Geometry: final body of the model. Coordinates: model frame, mm. A direction names the side the tool comes from. Coordinates: 2 decimals unless noted, no trailing zeros. Write each loop counter-clockwise with the first axis right and the second up, starting at its lowest first coordinate (ties: lowest second). Pieces come first, ordered by that corner, then holes. Notation, with made-up numbers: (-5.75, -30) -> (38.25, -30) arc R19 ccw to (38.25, 3) -> close; hole circle Ø10 at (71.5, 15). An arc over 180 degrees is marked (long way). One line per item, written item: value.
```python
from build123d import *

# Parameters (mm, degrees)
F1_DEPTH = 6
F2_SIZE  = 1
F3_W     = 12
F3_H     = 23
F4_DEPTH = 1
F5_COUNT = 4
F6_R     = 1
F7_DEPTH = 25


with BuildPart() as f1:
    # F0 (on Top) → F1 (new body)
    with BuildSketch(Plane.XY):
        with BuildLine():
            Line((11.3636297451, -30.5553255426), (-11.5303793462, 30.4927918061))
            ThreePointArc((-11.5303793462, 30.4927918061), (-30.524172541, -11.4470472475), (11.3636297451, -30.5553255426))
        make_face()
        with BuildLine():
            ThreePointArc((11.3636297451, -30.5553255426), (26.7695193241, -18.6051830186), (32.6, 0))
            ThreePointArc((32.6, 0), (18.5319944058, 26.8202383163), (-11.5303793462, 30.4927918061))
            Line((-11.5303793462, 30.4927918061), (11.3636297451, -30.5553255426))
        make_face()
    extrude(amount=F1_DEPTH)

    # F2
    f2_edges = [f1.edges().sort_by_distance(p)[0] for p in [
        (-11.36363, 30.555326, 6),
        (-11.36363, 30.555326, 0),
    ]]
    chamfer(f2_edges, length=F2_SIZE)

    # F3 (on Front) → F4 (join, symmetric)
    with BuildSketch(Plane.XZ):
        with Locations((-26.536149025, 14.6011034735)):
            Rectangle(F3_W, F3_H)
    extrude(amount=F4_DEPTH, both=True)

    # F5: F1 ×4 about axis
    f5_axis = Axis((0, 0, 5), (0, 0, -1))


with BuildPart() as f1_1:
    add(f1.part)
    for i in range(1, F5_COUNT):
        add(f1.part.rotate(f5_axis, i * 360 / F5_COUNT))

    # F6 (on Top) → F7 (cut)
    with BuildSketch(Plane.XY):
        with Locations((-29.5159034431, -2.5976577308)):
            Circle(F6_R)
        with Locations((29.5159034431, 2.5976577308)):
            Circle(F6_R)
    extrude(amount=F7_DEPTH, mode=Mode.SUBTRACT)


solid = f1_1.part
```
(1) Section B-B (y = 0). Return the cut outline in (x, z).
Responses:
outline: (-32.6, 1) -> (-31.6, 0) -> (31.6, 0) -> (32.6, 1) -> (32.6, 5) -> (32.54, 5.06) -> (32.54, 26.1) -> (20.54, 26.1) -> (20.54, 6) -> (-20.54, 6) -> (-20.54, 26.1) -> (-32.54, 26.1) -> (-32.54, 5.06) -> (-32.6, 5) -> close
(2) Pull-direction query (X, two-part tool) for faces 1 (the flat face through (-27, 0, 26.101)), 2 (the flat face through (1, 27, 16)), 3 (the flat face through (-20.536, 0, 16)); classes: released by +X, released by -X, zero draft, split by the parting line, or undercut.
Responses:
face 1: zero draft
face 2: released by +X
face 3: undercut
(3) Reachability of faces 4 (the flat face through (0, 27, 26.101)), 5 (the flat face through (0, 32.536, 15)), 6 (the flat face through (0, 0, 0)), 7 (the flat face through (32.536, 0, 15)), 8 (the flat face through (0, 20.536, 16)) from +Z, -Z, +X, -X, +Y, -Y: full face, straight path, thin tool, end or side. Return the list, or none.
Responses:
face 4: +Z, +X, -X, +Y, -Y
face 5: +Z, +X, -X, +Y
face 6: -Z, +X, -X, +Y, -Y
face 7: +Z, +X, +Y, -Y
face 8: +Z, +X, -X
(4) Line query: line 1 (Z direction, x = -3, y = 19); line 2 (X direction, y = -27, z = 12.75). Output: solid intervals per line, ascending. Write a range as [from, to].
Responses:
line 1: z = [0, 6]
line 2: x = [-1, 1]
(5) Section A-A (z = 9). Return the cut outline in (x, y), then the cut area to 3 significant figures.
Responses:
outline: (-32.54, -1) -> (-20.54, -1) -> (-20.54, 1) -> (-32.54, 1) -> close; (-1, -32.54) -> (1, -32.54) -> (1, -20.54) -> (-1, -20.54) -> close; (-1, 20.54) -> (1, 20.54) -> (1, 32.54) -> (-1, 32.54) -> close; (20.54, -1) -> (32.54, -1) -> (32.54, 1) -> (20.54, 1) -> close
area: 96.0 mm2
(6) First-contact query: pin 1 (2 mm diameter, centred on x = 5, z = 3.5, fed in from +Y); pin 2 (9.5 mm diameter, centred on y = -27, z = 14, fed in from +X); pin 3 (8 mm diameter, centred on x = -20, z = 11.5, fed in from +Y); pin 4 (1.2 mm diameter, centred on x = 29.52, y = 2.6, fed in from +Z). Flat tips, straight axial feed; report the tip coordinate or a pass-through.
Responses:
pin 1: stops at y = 32.35
pin 2: stops at x = 1
pin 3: stops at y = 1
pin 4: passes through
(7) Section C-C (z = 2.5). Return the cut outline in (x, y), then the cut area to 3 significant figures.
Responses:
outline: circle Ø65.2 at (0, 0); hole circle Ø2 at (-29.52, -2.6); hole circle Ø2 at (29.52, 2.6)
area: 3,330 mm2
